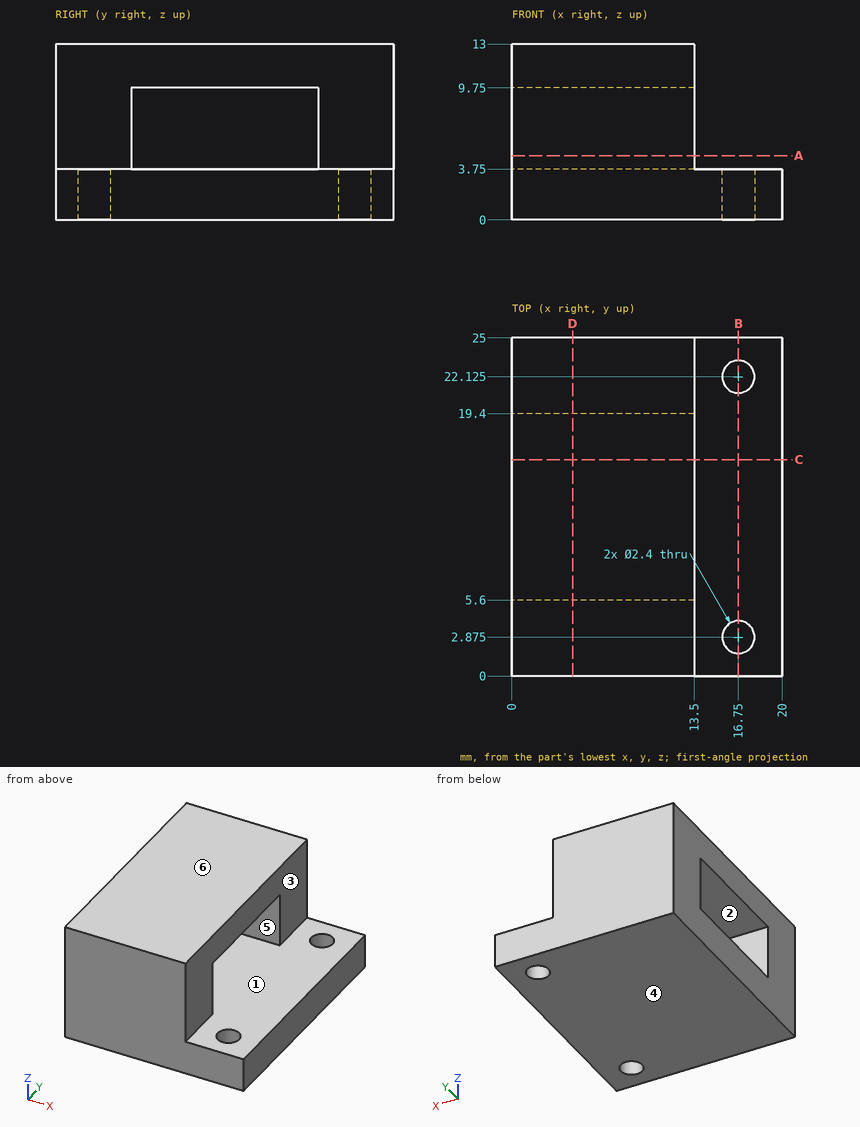
Design review of the part shown in the three views and the two pictorial views. Dimensions are in mm from the part's minimum x, y and z. A direction names the side the tool comes from. Round coordinates to 2 decimals unless told otherwise and drop trailing zeros. Loops run counter-clockwise (first coordinate to the right, second up) from the corner with the lowest first, then second, coordinate; pieces in that order, holes last.
(1) Tool access review of the marked faces 1, 2 and 3: name each direction out of +Z, -Z, +X, -X, +Y, -Y from which nothing blocks a thin tool from reaching the whole face with its end or side.
Returned:
face 1: +X
face 2: +X, -X
face 3: +Z, +X, +Y, -Y
(2) Wall thickness on line 1 along Y through (x, z) = (16.75, 1.3) (3 decimals); line 2 along Z through (x, y) = (3.25, 19); line 3 along X through (y, z) = (24.25, 4.5): over which ranges is each line inside the solid? List them lowest first.
Returned:
line 1: y = 0 to 1.675, 4.075 to 20.925, 23.325 to 25
line 2: z = 0 to 3.75, 9.75 to 13
line 3: x = 0 to 13.5
(3) Clearance check with flat-ended pins moving along their axes: P1, Ø3, axis at y = 7.5, z = 10, coming from the +X side; P2, Ø2, axis at x = 16.75, y = 22.125, coming from the -Z side. State where each tip first meets the part, or that it passes through.
Returned:
P1: stops at x = 13.5
P2: passes through
(4) We need section B-B (x = 16.75). Give the boundary of the cut face in (y, z) (3 decimals), plus the area to 4 significant figures.
Returned:
outline: (0, 0) - (1.675, 0) - (1.675, 3.75) - (0, 3.75) - close; (4.075, 0) - (20.925, 0) - (20.925, 3.75) - (4.075, 3.75) - close; (23.325, 0) - (25, 0) - (25, 3.75) - (23.325, 3.75) - close
area: 75.75 mm2
(5) We need section C-C (y = 16). Give the boundary of the cut face in (x, z).
Returned:
outline: (0, 0) - (20, 0) - (20, 3.75) - (0, 3.75) - close; (0, 9.75) - (13.5, 9.75) - (13.5, 13) - (0, 13) - close
(6) Mouldability with a two-part tool opening along Z and no side actions: class the marked faces 4, 5 and 6 as released by +Z, released by -Z, zero draft, split by the parting line, or undercut.
Returned:
face 4: released by -Z
face 5: undercut
face 6: released by +Z
(7) We need section A-A (z = 4.75). Give the boundary of the cut face in (x, y), plus the area to 3 significant figures.
Returned:
outline: (0, 0) - (13.5, 0) - (13.5, 5.6) - (0, 5.6) - close; (0, 19.4) - (13.5, 19.4) - (13.5, 25) - (0, 25) - close
area: 151 mm2
(8) We need section D-D (x = 4.5). Give the boundary of the cut face in (y, z).
Returned:
outline: (0, 0) - (25, 0) - (25, 13) - (0, 13) - close; hole (5.6, 3.75) - (19.4, 3.75) - (19.4, 9.75) - (5.6, 9.75) - close
